Read the model definition and answer for the solid it produces. Units are mm, in the model's axes. Coordinates: 2 decimals unless noted, no trailing zeros. Order: outer loops, then holes, each group sorted by start corner. A loop starts at its lowest first (then second) coordinate and runs counter-clockwise, first axis right, second up. Notation, with made-up numbers: (13.25, 2) - (29.25, 2) arc R21 cw to (29.25, 14) - close; hole circle Ø9 at (34, 83). An arc over 180 degrees is marked (long way). Use one line per item in the form item = value.
```python
from build123d import *

# Parameters (mm, degrees)
BOSS_EXTRUDE1_DEPTH = 3


with BuildPart() as part:
    # Sketch1 → Boss-Extrude1 (new body)
    with BuildSketch(Plane.XY):
        with BuildLine():
            Line((25, 0), (263, 0))
            ThreePointArc((263, 0), (280.67766953, 7.32233047), (288, 25))
            Line((288, 25), (288, 263))
            ThreePointArc((288, 263), (280.67766953, 280.67766953), (263, 288))
            Line((263, 288), (25, 288))
            ThreePointArc((25, 288), (7.32233047, 280.67766953), (0, 263))
            Line((0, 263), (0, 25))
            ThreePointArc((0, 25), (7.32233047, 7.32233047), (25, 0))
        make_face()
        with BuildLine():
            Line((25, 170), (113, 170))
            ThreePointArc((113, 170), (116.535533906, 171.464466094), (118, 175))
            Line((118, 175), (118, 263))
            ThreePointArc((118, 263), (116.535533906, 266.535533906), (113, 268))
            Line((113, 268), (25, 268))
            ThreePointArc((25, 268), (21.464466094, 266.535533906), (20, 263))
            Line((20, 263), (20, 175))
            ThreePointArc((20, 175), (21.464466094, 171.464466094), (25, 170))
        make_face(mode=Mode.SUBTRACT)
        with BuildLine():
            Line((118, 113), (118, 25))
            ThreePointArc((118, 25), (116.535533906, 21.464466094), (113, 20))
            Line((113, 20), (25, 20))
            ThreePointArc((25, 20), (21.464466094, 21.464466094), (20, 25))
            Line((20, 25), (20, 113))
            ThreePointArc((20, 113), (21.464466094, 116.535533906), (25, 118))
            Line((25, 118), (113, 118))
            ThreePointArc((113, 118), (116.535533906, 116.535533906), (118, 113))
        make_face(mode=Mode.SUBTRACT)
        with BuildLine():
            Line((263, 118), (175, 118))
            ThreePointArc((175, 118), (171.464466094, 116.535533906), (170, 113))
            Line((170, 113), (170, 25))
            ThreePointArc((170, 25), (171.464466094, 21.464466094), (175, 20))
            Line((175, 20), (263, 20))
            ThreePointArc((263, 20), (266.535533906, 21.464466094), (268, 25))
            Line((268, 25), (268, 113))
            ThreePointArc((268, 113), (266.535533906, 116.535533906), (263, 118))
        make_face(mode=Mode.SUBTRACT)
        with BuildLine():
            Line((170, 175), (170, 263))
            ThreePointArc((170, 263), (171.464466094, 266.535533906), (175, 268))
            Line((175, 268), (263, 268))
            ThreePointArc((263, 268), (266.535533906, 266.535533906), (268, 263))
            Line((268, 263), (268, 175))
            ThreePointArc((268, 175), (266.535533906, 171.464466094), (263, 170))
            Line((263, 170), (175, 170))
            ThreePointArc((175, 170), (171.464466094, 171.464466094), (170, 175))
        make_face(mode=Mode.SUBTRACT)
    extrude(amount=BOSS_EXTRUDE1_DEPTH)


solid = part.part
```
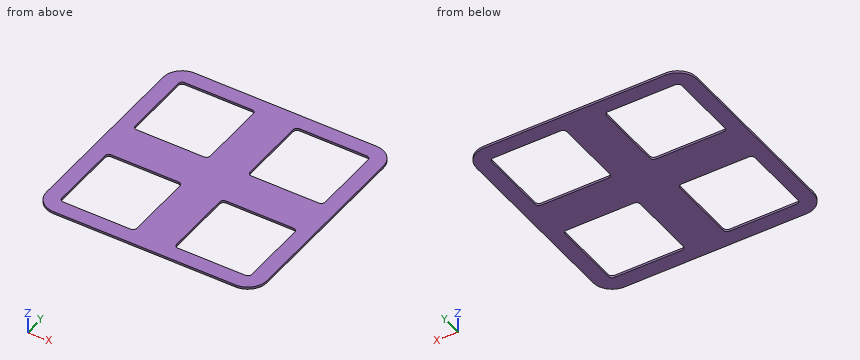
(1) Straight lines are drawn through the part: L1, parallel to Y at x = 229.5, z = 1.4; L2, parallel to X at y = 114, z = 1.8. For each, find the intervals that lie inside material, in ascending order.
Answer list:
L1 = 0 to 20, 118 to 170, 268 to 288
L2 = 0 to 20.1, 117.9 to 170.1, 267.9 to 288
(2) Section C-C, the plane z = 0.85 is taken. State how many separate pieces and enclosed holes the cut face has, then the cut area to 3 significant figures.
Answer list:
separate_pieces = 1
enclosed_holes = 4
area = 44,100 mm2
(3) Section A-A, the plane x = 183.5 is taken. Write down the section's boundary in (y, z), then the cut area to 3 significant figures.
Answer list:
outline = (0, 0) - (20, 0) - (20, 3) - (0, 3) - close; (118, 0) - (170, 0) - (170, 3) - (118, 3) - close; (268, 0) - (288, 0) - (288, 3) - (268, 3) - close
area = 276 mm2
